Solid Edge part; units mm, degrees
sketch "Sketch1" plane through (0, 0, 0) normal (0, 0, 1) x (1, 0, 0)
  line L0 (-28.575, 0) -> (28.575, 0)
  line L1 (28.575, 0) -> (28.575, 24.638)
  line L2 (28.575, 24.638) -> (-28.575, 24.638)
  line L3 (-28.575, 24.638) -> (-28.575, 0)
  dimension "D1" = 28.575
  dimension "D2" = 28.575
extrude "Protrusion1" add sketch "Sketch1" along normal blind 40.386
sketch "Sketch2" plane through (0, 12.319, 0) normal (0, 0, -1) x (1, 0, 0)
  circle A0 centre (-9.525, 1.905) radius 4.7625
extrude "ExtrudedProtrusion_2" add sketch "Sketch2" along normal blind 7.62
sketch "Sketch3" plane through (0, 0, 20.193) normal (0, -1, 0) x (1, 0, 0)
  line L0 (-28.575, 20.193) -> (-19.685, 20.193)
  line L1 (-19.685, 20.193) -> (-19.685, -7.747)
  line L2 (-19.685, -7.747) -> (-28.575, -7.747)
  line L3 (-28.575, -7.747) -> (-28.575, 20.193)
  dimension "D1" = 28.575
  dimension "D2" = 19.685
extrude "ExtrudedCutout_1" cut sketch "Sketch3" against normal blind 23.114
mirror "Mirror1" about plane through (0, 0, 0) normal (1, 0, 0) of "ExtrudedCutout_1"
hole "Hole_1" at (-24.765, 23.114, 17.526) direction (0, 1, 0) diameter 4.445 end up to next
hole "Hole1" at (24.765, 23.114, 17.526) direction (0, 1, 0) diameter 4.445 end up to next
hole "Hole2" at (24.765, 23.114, 27.686) direction (0, 1, 0) diameter 4.445 end up to next
hole "Hole3" at (-24.765, 23.114, 27.686) direction (0, 1, 0) diameter 4.445 end up to next
CAD build for the part. Positions are in the model's coordinates, mm. A direction names the side the tool comes from. Round coordinates to 2 decimals unless told otherwise and drop trailing zeros. Order: outer loops, then holes, each group sorted by start corner. A loop starts at its lowest first (then second) coordinate and runs counter-clockwise, first axis right, second up. Notation, with made-up numbers: (33, 70) -> (43, 70) arc R16 ccw to (43, 100) -> close; hole circle Ø10 at (-6.5, 36). An arc over 180 degrees is marked (long way). Write each question's results on one line, items separated by ' | '.
1. Cut at B-B (z = 33). Give the cut face in (x, y) (3 decimals), plus the area to 3 significant figures.
Findings below:
outline: (-28.575, 23.114) -> (-19.685, 23.114) -> (-19.685, 0) -> (19.685, 0) -> (19.685, 23.114) -> (28.575, 23.114) -> (28.575, 24.638) -> (-28.575, 24.638) -> close | area: 997 mm²
2. 3-axis set-ups, long thin cutter, end or side, ignore diameter. For faces 1 (the face through (22, 23.114, 27)), 2 (the face through (-24, 11, 12.446)), 3 (the face through (0, 0, 20)): which of +Z, -Z, +X, -X, +Y, -Y reach the whole face in a straight line?
Findings below:
face 1: +Z, +X, -Y | face 2: +Z, -X, -Y | face 3: +Z, -Z, +X, -X, -Y
3. Cut at D-D (y = 7). Give the cut face in (x, z) (3 decimals), plus the area to 3 significant figures.
Findings below:
outline: (-28.575, 0) -> (-12.846, 0) -> (-12.846, -7.62) -> (-6.204, -7.62) -> (-6.204, 0) -> (28.575, 0) -> (28.575, 12.446) -> (19.685, 12.446) -> (19.685, 40.386) -> (-19.685, 40.386) -> (-19.685, 12.446) -> (-28.575, 12.446) -> close | area: 1,860 mm²
4. Pull direction X, two halves, no side cores. Call faces 4 (the face through (22.595, 23.865, 18.008)), 5 (the face through (0, 12, 40.386)), 6 (the face through (-10.557, 5.765, -3.757)): pulls with the +X half, pulls with the -X half, needs draft (parallel to the pull), parting line crosses it, or undercut.
Findings below:
face 4: undercut | face 5: needs draft | face 6: parting line crosses it
5. Cut at A-A (y = 17). Give the cut face in (x, z) (3 decimals), plus the area to 3 significant figures.
Findings below:
outline: (-28.575, 0) -> (28.575, 0) -> (28.575, 12.446) -> (19.685, 12.446) -> (19.685, 40.386) -> (-19.685, 40.386) -> (-19.685, 12.446) -> (-28.575, 12.446) -> close | area: 1,810 mm²
6. Wall check: line 1 along Z through (x, y) = (-10.5, 20.5); line 2 along Z through (x, y) = (22, 10.75); line 3 along X through (y, z) = (13.5, 26.5) (3 decimals). Give the ranges that are in metal, low to high. Write a range as [from, to].
Findings below:
line 1: z = [0, 40.39] | line 2: z = [0, 12.45] | line 3: x = [-19.685, 19.685]
7. Flat gauge pins, fed straight in: P1, Ø11.5, axis at y = 11, z = 25.5, coming from the +X side (3 decimals); P2, Ø11.5, axis at y = 9.5, z = 29, coming from the -X side (3 decimals); P3, Ø7, axis at x = 24.5, y = 15.5, coming from the +Z side. Where does each tip first touch, or does it go through?
Findings below:
P1: stops at x = 19.685 | P2: stops at x = -19.685 | P3: stops at z = 12.45
8. Cut at C-C (x = -2). Give the cut face in (y, z).
Findings below:
outline: (0, 0) -> (24.64, 0) -> (24.64, 40.39) -> (0, 40.39) -> close
